from build123d import *

# Parameters (mm, degrees)
SKETCH_R        = 1.7
PAD_DEPTH       = 13
SKETCH001_W     = 101.56
SKETCH001_H     = 98.03
POCKET_DEPTH    = 10
SKETCH002_R     = 3
POCKET001_DEPTH = 3.1
SKETCH003_W     = 18.8
SKETCH003_H     = 7.5
POCKET002_DEPTH = 11


with BuildPart() as part:
    # Sketch → Pad (new body)
    with BuildSketch(Plane.XY):
        with BuildLine():
            Line((0, -5), (0, -111.03))
            ThreePointArc((0, -111.03), (1.464466, -114.565534), (5, -116.03))
            Line((5, -116.03), (114.56, -116.03))
            ThreePointArc((114.56, -116.03), (118.095534, -114.565534), (119.56, -111.03))
            Line((119.56, -111.03), (119.56, -5))
            ThreePointArc((119.56, -5), (118.095534, -1.464466), (114.56, 0))
            Line((114.56, 0), (5, 0))
            ThreePointArc((5, 0), (1.464466, -1.464466), (0, -5))
        make_face()
        with Locations((5, -5)):
            Circle(SKETCH_R, mode=Mode.SUBTRACT)
        with Locations((114.56, -5)):
            Circle(SKETCH_R, mode=Mode.SUBTRACT)
        with Locations((114.56, -111.03)):
            Circle(SKETCH_R, mode=Mode.SUBTRACT)
        with Locations((5, -111.03)):
            Circle(SKETCH_R, mode=Mode.SUBTRACT)
    extrude(amount=-PAD_DEPTH)

    # Sketch001 → Pocket (cut)
    with BuildSketch(Plane.XY):
        with Locations((59.78, -58.015)):
            Rectangle(SKETCH001_W, SKETCH001_H)
    extrude(amount=-POCKET_DEPTH, mode=Mode.SUBTRACT)

    # Sketch002 (on Face5 of Pocket) → Pocket001 (cut)
    with BuildSketch(Plane(origin=(0, 0, -13), x_dir=(1, 0, 0), z_dir=(0, 0, -1))):
        with Locations((5, 111.03)):
            Circle(SKETCH002_R)
        with Locations((114.56, 111.03)):
            Circle(SKETCH002_R)
        with Locations((5, 5)):
            Circle(SKETCH002_R)
        with Locations((114.56, 5)):
            Circle(SKETCH002_R)
    extrude(amount=-POCKET001_DEPTH, mode=Mode.SUBTRACT)

    # Sketch003 → Pocket002 (cut)
    with BuildSketch(Plane.XZ):
        with Locations((37.81, -3.75)):
            Rectangle(SKETCH003_W, SKETCH003_H)
    extrude(amount=POCKET002_DEPTH, mode=Mode.SUBTRACT)


with BuildPart() as part_1:
    # Body001 placement: moved
    add(part.part.moved(Location((-16.22, 33.17, 0))))


solid = part_1.part
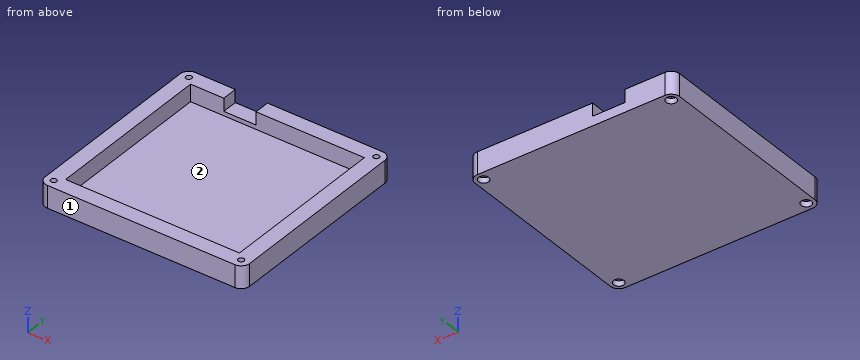
The model under review builds one solid part; all positions refer to its coordinate system, in mm. Face numbers are marked on the shaded views. A direction names the side the tool comes from. Round coordinates to 2 decimals unless told otherwise and drop trailing zeros. Write each loop counter-clockwise with the first axis right and the second up, starting at its lowest first coordinate (ties: lowest second). Pieces come first, ordered by that corner, then holes. Notation, with made-up numbers: M 4,3.25 L 37,3.25 A32 cw 37,39.25 Z; hole C 85,-29.75 d10. An arc over 180 degrees is marked long. Answer as CSV lines item,"result". Start each with the question number.
Q1. Clearance check with flat-ended pins moving along their axes: P1, Ø2, axis at x = -11.22, y = -77.86, coming from the -Z side; P2, Ø5, axis at x = 98.34, y = 28.17, coming from the +Z side; P3, Ø4.5, axis at x = 24.5, y = 29, coming from the +Z side; P4, Ø4, axis at x = -11.22, y = 28.17, coming from the -Z side. State where each tip first meets the part, or that it passes through.
Q2. Consider section C-C, the plane y = -33.5. Give the boundary of the cut face in (x, z).
Q3. Consider section B-B, the plane x = 80. Give the boundary of the cut face in (y, z), then the cut area to 3 significant figures.
Q4. Consider section A-A, the plane z = -1.75. Give the boundary of the cut face in (x, y), then the cut area to 3 significant figures.
Q5. Tool access review of the marked faces 1 and 2: name each direction out of +Z, -Z, +X, -X, +Y, -Y from which nothing blocks a thin tool from reaching the whole face with its end or side.
Q6. Wall thickness on line 1 along X through (y, z) = (-77.86, -10.7); line 2 along X through (y, z) = (-77.86, -5.25); line 3 along Y through (x, z) = (98.34, -11.2): over which ranges is each line inside the solid? List them lowest first.
Result set:
1,P1,"passes through"
1,P2,"stops at z = 0"
1,P3,"stops at z = -7.5"
1,P4,"stops at z = -9.9"
2,outline,"M -16.22,-13 L 103.34,-13 L 103.34,0 L 94.34,0 L 94.34,-10 L -7.22,-10 L -7.22,0 L -16.22,0 Z"
3,outline,"M -82.86,-13 L 33.17,-13 L 33.17,0 L 24.17,0 L 24.17,-10 L -73.86,-10 L -73.86,0 L -82.86,0 Z"
3,area,"528 mm²"
4,outline,"M -16.22,-77.86 A5 ccw -11.22,-82.86 L 98.34,-82.86 A5 ccw 103.34,-77.86 L 103.34,28.17 A5 ccw 98.34,33.17 L 30.99,33.17 L 30.99,24.17 L 94.34,24.17 L 94.34,-73.86 L -7.22,-73.86 L -7.22,24.17 L 12.19,24.17 L 12.19,33.17 L -11.22,33.17 A5 ccw -16.22,28.17 Z; hole C -11.22,-77.86 d3.4; hole C -11.22,28.17 d3.4; hole C 98.34,-77.86 d3.4; hole C 98.34,28.17 d3.4"
4,area,"3,690 mm²"
5,face 1,"+Z, -Z, +X, -X, -Y"
5,face 2,"+Z"
6,line 1,"x = -16.22 to -14.22, -8.22 to 95.34, 101.34 to 103.34"
6,line 2,"x = -16.22 to -12.92, -9.52 to 96.64, 100.04 to 103.34"
6,line 3,"y = -82.86 to -80.86, -74.86 to 25.17, 31.17 to 33.17"
